The model under review builds one solid part; all positions refer to its coordinate system, in mm. A direction names the side the tool comes from. Coordinates: 2 decimals unless noted, no trailing zeros. Order: outer loops, then holes, each group sorted by start corner. A loop starts at its lowest first (then second) coordinate and runs counter-clockwise, first axis right, second up. Notation, with made-up numbers: (68, 27.5) - (82, 27.5) arc R23 cw to (82, 44.5) - close; hole circle Ø1 at (24, 74.25). An arc over 180 degrees is marked (long way). Answer in a Markdown table with one row per item.
Autodesk Inventor part; units mm, degrees
ref_plane "YZ Plane" through (0, 0, 0) normal (1, 0, 0) x (0, 1, 0)
ref_plane "XZ Plane" through (0, 0, 0) normal (0, 1, 0) x (-1, 0, 0)
ref_plane "XY Plane" through (0, 0, 0) normal (0, 0, 1) x (1, 0, 0)
sketch "Sketch1" plane through (0, 0, 0) normal (0, 1, 0) x (-1, 0, 0)
  line L0 (0, 0) -> (-29.7815, 0)
  line L1 (-29.7815, 0) -> (-29.7815, -37.2745)
  line L2 (-29.7815, -37.2745) -> (0, -37.2745)
  line L3 (0, -37.2745) -> (0, 0)
  line L4 (-14.8907, -37.2745) -> (-14.8907, 0)
  line L5 (0, -18.6373) -> (-29.7815, -18.6373)
  circle A0 centre (-14.8907, -18.6373) radius 10.8903
  dimension "d0" = 29.7815
  dimension "d1" = 37.2745
  dimension "d2" = 21.7805
extrude "Extrusion1" add sketch "Sketch1" against normal blind 34
extrude "Extrusion2" add sketch "Sketch1" along normal blind 1 contours A0 L5 L4 | L4 L5 A0 | A0 L4 L5 | L4 A0 L5
sketch "Sketch2" plane through (14.8907, 1, -18.6373) normal (0, 1, 0) x (1, 0, 0)
  circle A0 centre (0, 0) radius 12
  dimension "d9" = 24
extrude "Extrusion3" add sketch "Sketch2" along normal blind 7.5
sketch "Sketch3" plane through (14.8907, 8.5, -18.6373) normal (0, 1, 0) x (1, 0, 0)
  circle A0 centre (0, 0) radius 10.925
  circle A1 centre (0, 0) radius 12
  line L0 (-3.175, -12) -> (3.175, -12)
  line L1 (3.175, -12) -> (3.175, 12)
  line L2 (3.175, 12) -> (-3.175, 12)
  line L3 (-3.175, 12) -> (-3.175, -12)
  line L4 (-3.175, -12) -> (3.175, 12) construction
  line L5 (3.175, -12) -> (-3.175, 12) construction
  point P0 (-3.175, -11.5724)
  point P1 (3.175, -11.5724)
  point P2 (-3.175, 11.5724)
  point P3 (3.175, 11.5724)
  point P4 (0, -12)
  point P5 (0, 12)
  point P6 (-3.175, -10.4535)
  point P7 (3.175, -10.4535)
  dimension "d12" = 21.85
  dimension "d21" = 6.35
extrude "Extrusion4" add sketch "Sketch3" along normal blind 10 contours A0 L1 | L1 A0 L3 | L3 A0
thread "Thread2"
thread "Thread3"
extrude "Extrusion5" cut sketch "Sketch3" against normal up to surface (7.5 mm away) contours L1 A1 L3 A0 picked at (0, -11.2482)
sketch "Sketch4" plane through (14.8907, 18.5, -18.6373) normal (0, 1, 0) x (1, 0, 0)
  circle A0 centre (0, 0) radius 10.925
  line L0 (-1.75, 10.925) -> (1.75, 10.925)
  line L1 (1.75, 10.925) -> (1.75, -10.925)
  line L2 (1.75, -10.925) -> (-1.75, -10.925)
  line L3 (-1.75, -10.925) -> (-1.75, 10.925)
  line L4 (-1.75, 10.925) -> (1.75, -10.925) construction
  line L5 (1.75, 10.925) -> (-1.75, -10.925) construction
  circle A1 centre (0, 0) radius 10
  line L6 (-10.925, -1.75) -> (10.925, -1.75)
  line L7 (10.925, -1.75) -> (10.925, 1.75)
  line L8 (10.925, 1.75) -> (-10.925, 1.75)
  line L9 (-10.925, 1.75) -> (-10.925, -1.75)
  line L10 (-10.925, -1.75) -> (10.925, 1.75) construction
  line L11 (10.925, -1.75) -> (-10.925, 1.75) construction
  point P0 (-9.8457, 1.75)
  point P1 (-10.7839, 1.75)
  point P2 (-10.7839, -1.75)
  point P3 (-9.8457, -1.75)
  point P4 (-1.75, 9.8457)
  point P5 (1.75, 9.8457)
  point P6 (1.75, 10.7839)
  point P7 (-1.75, 10.7839)
  point P8 (10.7839, 1.75)
  point P9 (9.8457, 1.75)
  point P10 (9.8457, -1.75)
  point P11 (10.7839, -1.75)
  point P12 (1.75, -9.8457)
  point P13 (-1.75, -9.8457)
  point P14 (-1.75, -10.7839)
  point P15 (1.75, -10.7839)
  dimension "d25" = 3.5
  dimension "d26" = 20
  dimension "d27" = 3.5
extrude "Extrusion6" cut sketch "Sketch4" against normal blind 6 contours A0 L6 A1 L8 | L1 A1 L3 A0 | A0 L3 A1 L1 | L8 A1 L6 A0
hole "Hole1" at (14.8907, 18.5, -18.6373) direction (0, -1, 0) diameter 18.5 depth 18.5
properties material "ABS Plastic"
Item 1: To check wall thickness, follow line 1 (Z direction, x = 14.75, y = 7); line 2 (Y direction, x = 28.75, z = -23); line 3 (Z direction, x = 20, y = 14). State the ranges of each line that lie inside material, in increasing order. Write a range as from..to.
Check values:
| item | result |
|---|---|
| line 1 | -30.64..-27.89, -9.39..-7.71 |
| line 2 | -34..0 |
| line 3 | -28.29..-26.35, -10.93..-8.98 |
Item 2: Mouldability with a two-part tool opening along X and no side actions: class faces 4 (the face through (0, -17, -19)), 5 (the face through (20.519, 9.12, -25.978)), 6 (the face through (15, 12.5, -29)), 7 (the face through (4.5, 12.5, -18.7)) as +X half, -X half, draft (parallel to the pull), parting line (faces both ways), or undercut.
Check values:
| item | result |
|---|---|
| face 4 | -X half |
| face 5 | undercut |
| face 6 | undercut |
| face 7 | draft |
Item 3: We need section D-D, the plane z = -33.5. Write out the cut boundary in (x, y), then the cut area to 3 significant figures.
Check values:
| item | result |
|---|---|
| outline | (0, -34) - (29.78, -34) - (29.78, 0) - (0, 0) - close |
| area | 1,010 mm^2 |
Item 4: Tool access review of faces 1 (the face through (9, 1, -28)), 2 (the face through (15, 12.5, -8)), 3 (the face through (14.408, 4.698, -30.628)): name each direction out of +Z, -Z, +X, -X, +Y, -Y from which nothing blocks a thin tool from reaching the whole face with its end or side.
Check values:
| item | result |
|---|---|
| face 1 | none |
| face 2 | +Z, +Y |
| face 3 | +Y |
Item 5: We need section A-A, the plane z = -22. Write out the cut boundary in (x, y), then the cut area to 3 significant figures.
Check values:
| item | result |
|---|---|
| outline | (0, -34) - (29.78, -34) - (29.78, 0) - (25.25, 0) - (25.25, 1) - (26.41, 1) - (26.41, 8.5) - (25.29, 8.5) - (25.29, 18.5) - (23.51, 18.5) - (23.51, 0) - (6.27, 0) - (6.27, 18.5) - (4.5, 18.5) - (4.5, 8.5) - (3.37, 8.5) - (3.37, 1) - (4.53, 1) - (4.53, 0) - (0, 0) - close |
| area | 1,100 mm^2 |
Item 6: Clearance check with flat-ended pins moving along their axes: pin 1 Ø1.2 at (x, z) = (15.5, -8) entering from +Y; pin 2 Ø10 at (x, y) = (11.5, 9) entering from -Z; pin 3 Ø1 at (x, y) = (4.5, 14.5) entering from +Z. State where each tip first meets the part, or that it passes through.
Check values:
| item | result |
|---|---|
| pin 1 | y = 12.5 |
| pin 2 | z = -30.64 |
| pin 3 | z = -14 |
Item 7: We need section B-B, the plane y = 5.5. Write out the cut boundary in (x, z) (3 decimals).
Check values:
| item | result |
|---|---|
| outline | (11.716, -8.184) - (11.716, -7.065) arc R12 ccw (long way) to (18.066, -7.065) - (18.066, -8.184) arc R10.925 ccw to start; hole circle Ø18.5 at (14.891, -18.637) |
Item 8: We need section C-C, the plane x = 19.5. Write out the cut boundary in (y, z).
Check values:
| item | result |
|---|---|
| outline | (-34, -37.27) - (0, -37.27) - (0, -28.5) - (1, -28.5) - (1, -29.72) - (8.5, -29.72) - (8.5, -28.54) - (18.5, -28.54) - (18.5, -26.66) - (0, -26.66) - (0, -10.62) - (18.5, -10.62) - (18.5, -8.73) - (8.5, -8.73) - (8.5, -7.56) - (1, -7.56) - (1, -8.77) - (0, -8.77) - (0, 0) - (-34, 0) - close |
